Could you check a few things on this model? Use its own coordinates, in mm. Face numbers are marked on the shaded views. Coordinates: 2 decimals unless noted, no trailing zeros. Order: outer loops, then holes, each group sorted by start corner. A loop starts at its lowest first (then second) coordinate and runs counter-clockwise, first axis right, second up. Notation, with made-up numbers: (53, -17.75) -> (89, -17.75) arc R13 cw to (89, -1.75) -> close; hole circle Ø7 at (75, -38). An arc over 180 degrees is marked (long way). Return JSON: item names as keys, results as strings. Group by question number.
Solid Edge part; units mm, degrees
sketch "Sketch1" plane through (0, 0, 0) normal (0, 0, 1) x (1, 0, 0)
  line L0 (-13.5, -17.1) -> (13.5, -17.1)
  line L1 (13.5, -17.1) -> (13.5, 17.1)
  line L2 (13.5, 17.1) -> (-13.5, 17.1)
  line L3 (-13.5, 17.1) -> (-13.5, -17.1)
  dimension "D1" = 13.5
  dimension "D2" = 13.5
extrude "Protrusion1" add sketch "Sketch1" along normal blind 4.7625
hole "Hole_1" at (-10, 10, 4.7625) direction (0, 0, -1) diameter 3.4 end up to next
pattern_linear "Pattern1" count 2 spacing 20 along (1, 0, 0) count 2 spacing 20 along (0, -1, 0) of "Hole_1"
fillet "Round_1" radius 5 4 edges at (-13.5, -17.1, 2.3812) (13.5, -17.1, 2.3812) (13.5, 17.1, 2.3812) (-13.5, 17.1, 2.3812)
properties material "Aluminum, 6061-T6"
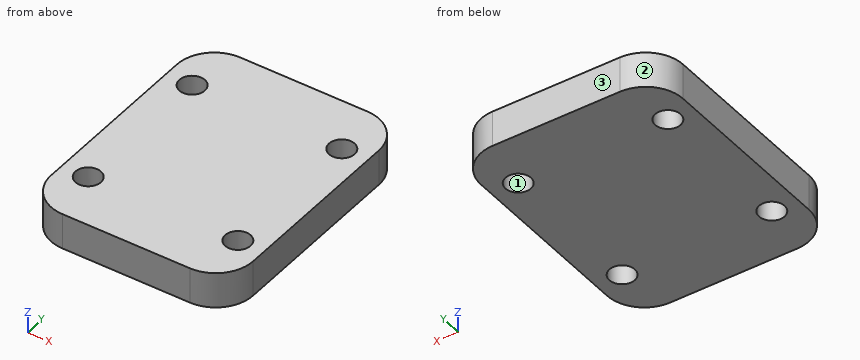
Q1. I want a section at B-B on z = 1.7. Please give me the cut outline in (x, y), and give its area (3 significant figures).
Q2. I'm going to push flat-ended pins straight in: pin 1 Ø2 at (x, y) = (-10, 10) entering from -Z; pin 2 Ø1 at (y, z) = (13, 1.5) entering from -X. Where does each tip first touch, or does it pass through?
Q3. We'd pull the mould along X, two halves only. Please class the marked faces 1, 2 and 3: pulls with the +X half, pulls with the -X half, needs draft (parallel to the pull), parting line crosses it, or undercut.
Q4. I want a section at C-C on x = -10. Please give me the cut outline in (y, z).
Q5. I need wall thicknesses on line 1 along X through (y, z) = (10, 2); line 2 along Y through (x, z) = (10, 2.4); line 3 along X through (y, z) = (-11.5, 2.15). Which ranges of each line are inside material? Lowest first, please. Write a range as from..to.
Q6. I want a section at A-A on y = 10. Please give me the cut outline in (x, z), and give its area (3 significant figures).
Response values:
{
 "1": {"outline": "(-13.5, -12.1) arc R5 ccw to (-8.5, -17.1) -> (8.5, -17.1) arc R5 ccw to (13.5, -12.1) -> (13.5, 12.1) arc R5 ccw to (8.5, 17.1) -> (-8.5, 17.1) arc R5 ccw to (-13.5, 12.1) -> close; hole circle Ø3.4 at (-10, -10); hole circle Ø3.4 at (-10, 10); hole circle Ø3.4 at (10, -10); hole circle Ø3.4 at (10, 10)", "area": "866 mm²"},
 "2": {"pin 1": "passes through", "pin 2": "stops at x = -13.48"},
 "3": {"face 1": "undercut", "face 2": "pulls with the -X half", "face 3": "needs draft"},
 "4": {"outline": "(-16.87, 0) -> (-11.7, 0) -> (-11.7, 4.76) -> (-16.87, 4.76) -> close; (-8.3, 0) -> (8.3, 0) -> (8.3, 4.76) -> (-8.3, 4.76) -> close; (11.7, 0) -> (16.87, 0) -> (16.87, 4.76) -> (11.7, 4.76) -> close"},
 "5": {"line 1": "x = -13.5..-11.7, -8.3..8.3, 11.7..13.5", "line 2": "y = -16.87..-11.7, -8.3..8.3, 11.7..16.87", "line 3": "x = -13.5..-10.8, -9.2..9.2, 10.8..13.5"},
 "6": {"outline": "(-13.5, 0) -> (-11.7, 0) -> (-11.7, 4.76) -> (-13.5, 4.76) -> close; (-8.3, 0) -> (8.3, 0) -> (8.3, 4.76) -> (-8.3, 4.76) -> close; (11.7, 0) -> (13.5, 0) -> (13.5, 4.76) -> (11.7, 4.76) -> close", "area": "96.2 mm²"}
}
